Autodesk Inventor part; units mm, degrees
ref_plane "YZ Plane" through (0, 0, 0) normal (1, 0, 0) x (0, 1, 0)
ref_plane "XZ Plane" through (0, 0, 0) normal (0, 1, 0) x (-1, 0, 0)
ref_plane "XY Plane" through (0, 0, 0) normal (0, 0, 1) x (1, 0, 0)
sketch "Sketch1" plane through (0, 0, 0) normal (0, 1, 0) x (-1, 0, 0)
  line L0 (0, 0) -> (-100, 0)
  line L1 (-100, 0) -> (-100, -25)
  line L2 (-100, -25) -> (0, -25)
  line L3 (0, -25) -> (0, 0)
  line L4 (-100, -25) -> (-75, -25)
  line L5 (-75, -25) -> (-75, -125)
  line L6 (-75, -125) -> (-100, -125)
  line L7 (-100, -125) -> (-100, -25)
  dimension "d0" = 100
  dimension "d1" = 25
  dimension "d2" = 25
  dimension "d3" = 100
extrude "Extrusion1" add sketch "Sketch1" along normal blind 2
sketch "Sketch2" plane through (0, 0, 0) normal (0, -1, 0) x (1, 0, 0)
  line L0 (100, 0) -> (100, -125)
  line L1 (75, -125) -> (75, -25)
  line L2 (100, -125) -> (75, -125)
  line L3 (75, -125) -> (75, -112.5)
  line L4 (75, -112.5) -> (100, -112.5)
  line L5 (100, -112.5) -> (100, -125)
  line L6 (88.5, -112.5) -> (86.5, -112.5)
  line L7 (86.5, -112.5) -> (86.5, -11.5)
  line L8 (86.5, -11.5) -> (88.5, -11.5)
  line L9 (88.5, -11.5) -> (88.5, -112.5)
  line L10 (86.5, -11.5) -> (46.5, -11.5)
  line L11 (46.5, -11.5) -> (46.5, -13.5)
  line L12 (46.5, -13.5) -> (86.5, -13.5)
  line L13 (86.5, -13.5) -> (86.5, -11.5)
  line L14 (0, 0) -> (100, 0)
  line L15 (75, -25) -> (0, -25)
  line L16 (46.5, 0) -> (36.5, 0)
  line L17 (36.5, 0) -> (36.5, -25)
  line L18 (36.5, -25) -> (46.5, -25)
  line L19 (46.5, -25) -> (46.5, 0)
  dimension "d6" = 12.5
  dimension "d7" = 101
  dimension "d8" = 2
  dimension "d9" = 11.5
  dimension "d10" = 40
  dimension "d11" = 2
  dimension "d12" = 10
extrude "Extrusion2" add sketch "Sketch2" along normal blind 4 contours L19 L11 L15 L17 L14 | L4 L7 L8 L9 | L10 L7 L12 L11
extrude "Extrusion3" add sketch "Sketch2" along normal blind 15 contours L0 L2 L1 L4
sketch "Sketch3" plane through (0, -15, 0) normal (0, -1, 0) x (1, 0, 0)
  circle A0 centre (90.65, -122.4) radius 1.55
  circle A1 centre (84.35, -122.4) radius 1.55
  line L0 (75, -125) -> (100, -125)
  line L1 (75, -112.5) -> (75, -125)
  point P0 (0, 0)
  dimension "d17" = 3.1
  dimension "d18" = 3.1
  dimension "d19" = 2.6
  dimension "d20" = 2.6
  dimension "d21" = 6.3
  dimension "d22" = 9.35
extrude "Extrusion4" add sketch "Sketch3" along normal blind 3
sketch "Sketch4" plane through (0, -4, 0) normal (0, -1, 0) x (1, 0, 0)
  line L0 (46.5, -11.5) -> (46.5, 0)
  line L1 (36.5, -25) -> (36.5, 0)
  line L2 (46.5, 0) -> (36.5, 0)
  line L3 (36.5, 0) -> (36.5, -6)
  line L4 (36.5, -6) -> (46.5, -6)
  line L5 (46.5, -6) -> (46.5, 0)
  line L6 (46.5, -13.5) -> (46.5, -25)
  line L7 (46.5, -25) -> (36.5, -25)
  line L8 (36.5, -25) -> (36.5, -19)
  line L9 (36.5, -19) -> (46.5, -19)
  line L10 (46.5, -19) -> (46.5, -25)
  point P0 (0, 0)
  point P1 (41.5, 0)
  dimension "d25" = 6
  dimension "d26" = 6
extrude "Extrusion5" cut sketch "Sketch4" against normal blind 2
sketch "Sketch5" plane through (86.5, -4, -13.5) normal (-1, 0, 0) x (0, 0, 1)
  line L0 (-99, 4) -> (-11.5, 4)
  line L1 (-25.7317, 4) -> (-30.7317, 4)
  line L2 (-30.7317, 4) -> (-30.7317, 2.5)
  line L3 (-30.7317, 2.5) -> (-25.7317, 2.5)
  line L4 (-25.7317, 2.5) -> (-25.7317, 4)
  point P0 (13.5, 4)
  dimension "d29" = 5
  dimension "d30" = 1.5
extrude "Extrusion6" cut sketch "Sketch5" against normal blind 2
sketch "Sketch6" plane through (86.5, 0, -13.5) normal (0, 0, -1) x (-1, 0, 0)
  line L0 (11.5, 0) -> (40, 0)
  line L1 (21.6385, 0) -> (16.6385, 0)
  line L2 (16.6385, 0) -> (16.6385, -1.5)
  line L3 (16.6385, -1.5) -> (21.6385, -1.5)
  line L4 (21.6385, -1.5) -> (21.6385, 0)
  point P0 (86.5, 0)
  point P1 (16.6385, 0)
  dimension "d33" = 5
  dimension "d34" = 1.5
extrude "Extrusion7" cut sketch "Sketch6" against normal blind 2
fillet "Fillet1" radius 4 5 edges at (100, -6.5, -125) (100, -7.5, -112.5) (75, -6.5, -125) (75, -7.5, -112.5) (87.5, 2, -125)
fillet "Fillet2" radius 35 1 edges at (100, 1, 0)
fillet "Fillet2" radius 10 1 edges at (75, 1, -25)
fillet "Fillet2" radius 23.5 1 edges at (88.5, -2, -11.5)
fillet "Fillet2" radius 21.5 1 edges at (86.5, -2, -13.5)
sketch "Sketch7" plane through (0, 0, 0) normal (0, -1, 0) x (1, 0, 0)
  line L0 (0, -25) -> (0, 0)
  line L1 (36.5, -25) -> (0, -25)
  point P0 (4, -12.5)
  dimension "d42" = 4
  dimension "d43" = 12.5
hole "Hole1" at (4, 0, -12.5) direction (0, 1, 0) diameter 3.2 end through all
equation "\"d20\" = d19"
properties part number "mlx_holder"
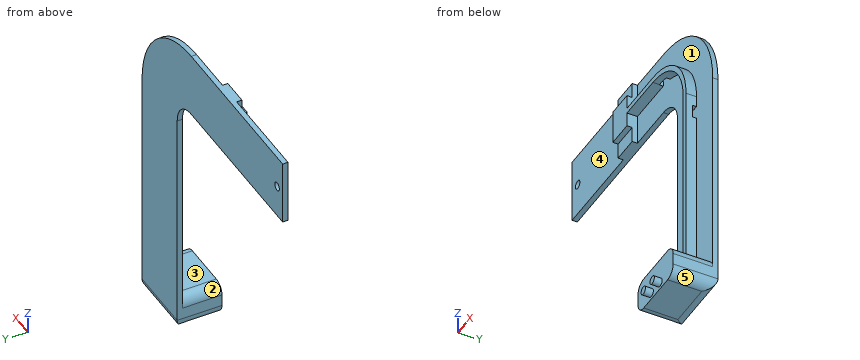
Read the model definition and answer for the solid it produces. Units are mm, in the model's axes. Face numbers are marked on the shaded views. A direction names the side the tool comes from. Round coordinates to 2 decimals unless told otherwise and drop trailing zeros. Write each loop counter-clockwise with the first axis right and the second up, starting at its lowest first coordinate (ties: lowest second). Pieces come first, ordered by that corner, then holes.
1. Determine the mould class of the marked faces 1, 2 and 3 for opening direction X: pulls with the +X half, pulls with the -X half, needs draft (parallel to the pull), parting line crosses it, or undercut.
2. Straight lines are drawn through the part: L1, parallel to Z at x = 4, y = 0.65; L2, parallel to Y at x = 75.5, z = -48.5; L3, parallel to X at y = 0.85, z = -12.5. For each, find the intervals that lie inside material, in ascending order.
3. The part is cut by section C-C, the plane x = 40.5. Determine the outline of the cut face in (y, z), then the cut area to 3 significant figures.
4. The part is cut by section A-A, the plane x = 4. Determine the outline of the cut face in (y, z).
5. Given pin 1 Ø1.2 at (x, y) = (87.5, -1) entering from -Z; pin 2 Ø4 at (x, z) = (87, -62.5) entering from -Y; pin 3 Ø4.5 at (y, z) = (-2, -17.5) entering from -X; pin 4 Ø4 at (x, z) = (91.5, -116.5) entering from -Y, each flat-ended and moving along its own axis, determine where each tip first touches the part or whether it passes through.
6. Which of the six approach directions +Z, -Z, +X, -X, +Y, -Y give full straight-line access (tool end or side, diameter ignored) to the marked faces 4 and 5?
7. The part is cut by section B-B, the plane y = -11.75. Determine the outline of the cut face in (x, z).
8. The part is cut by section D-D, the plane z = -122.4. Determine the outline of the cut face in (x, y).
Values:
1. face 1: undercut
1. face 2: pulls with the -X half
1. face 3: needs draft
2. L1: z = -25 to -14.1, -10.9 to 0
2. L2: y = 0 to 2
2. L3: x = 0 to 2.4, 5.6 to 91.81
3. outline: (-4, -19) - (-2, -19) - (-2, -25) - (2, -25) - (2, 0) - (-2, 0) - (-2, -6) - (-4, -6) - close
3. area: 126 mm2
4. outline: (0, -25) - (2, -25) - (2, -14.1) - (0, -14.1) - close; (0, -10.9) - (2, -10.9) - (2, 0) - (0, 0) - close
5. pin 1: stops at z = -124.98
5. pin 2: stops at y = -4
5. pin 3: stops at x = 0
5. pin 4: stops at y = -15
6. face 4: +Z, -Z, -X, -Y
6. face 5: -Z, +X, +Y, -Y
7. outline: (75, -121) arc R4 ccw to (79, -125) - (96, -125) arc R4 ccw to (100, -121) - (100, -116.5) arc R4 ccw to (96, -112.5) - (79, -112.5) arc R4 ccw to (75, -116.5) - close
8. outline: (75.25, -15) - (82.8, -15) - (82.8, -18) - (85.9, -18) - (85.9, -15) - (89.1, -15) - (89.1, -18) - (92.2, -18) - (92.2, -15) - (99.75, -15) - (99.75, 1.75) - (75.25, 1.75) - close
